Could you check a few things on this model? Use its own coordinates, in mm. A direction names the side the tool comes from. Give positions to 0.01 mm unless a question says otherwise; leave off trailing zeros. Write each loop counter-clockwise with the first axis right and the second up, starting at its lowest first coordinate (ties: lowest second). Pieces come first, ordered by that corner, then holes. Notation, with made-up numbers: M 19,87.5 L 67,87.5 A18 ccw 67,121.5 Z; hole C 13.25,79.25 d5. An arc over 180 degrees is marked long. Answer as CSV lines item,"result". Start each with the question number.
from build123d import *

# Parameters (mm, degrees)
F0_W      = 89.74328
F0_H      = 89.74328
F1_DEPTH  = 112.649
F3_DEPTH  = 8.382
F5_DEPTH  = 10.16
F7_DEPTH  = 10.16
F9_DEPTH  = 25.4
F10_R     = 25.4
F11_DEPTH = 12.7
F12_R     = 19.05
F13_DEPTH = 12.7
F14_R     = 12.7
F15_DEPTH = 42.97172


# Not quite as in the source:
# - a fillet or chamfer that OpenCascade refuses, or shapes differently, is made with other operations: its cross-section is extruded or revolved along the edge and cut away or added


with BuildPart() as f1:
    # F0 (on Right) → F1 (new body)
    with BuildSketch(Plane.YZ):
        with Locations((-0.1941993833, -7.4997466138)):
            Rectangle(F0_W, F0_H)
    extrude(amount=F1_DEPTH)

    # F2 (on face) → F3 (cut)
    with BuildSketch(Plane.XZ.offset(45.0658393833)):
        with BuildLine():
            ThreePointArc((103.9495, 19.7087333862), (103.0195640303, 21.9537974165), (100.7745, 22.8837333862))
            Line((100.7745, 22.8837333862), (11.8745, 22.8837333862))
            ThreePointArc((11.8745, 22.8837333862), (9.6294359697, 21.9537974165), (8.6995, 19.7087333862))
            Line((8.6995, 19.7087333862), (8.6995, 5.9419333862))
            ThreePointArc((8.6995, 5.9419333862), (9.6294359697, 3.6968693559), (11.8745, 2.7669333862))
            Line((11.8745, 2.7669333862), (100.7745, 2.7669333862))
            ThreePointArc((100.7745, 2.7669333862), (103.0195640303, 3.6968693559), (103.9495, 5.9419333862))
            Line((103.9495, 5.9419333862), (103.9495, 19.7087333862))
        make_face()
    extrude(amount=-F3_DEPTH, mode=Mode.SUBTRACT)

    # F4 (on face) → F5 (cut)
    with BuildSketch(Plane.XZ.offset(36.6838393833)):
        with BuildLine():
            ThreePointArc((8.6995, 8.0628333862), (9.6294359697, 5.8177693559), (11.8745, 4.8878333862))
            Line((11.8745, 4.8878333862), (100.7745, 4.8878333862))
            ThreePointArc((100.7745, 4.8878333862), (103.0195640303, 5.8177693559), (103.9495, 8.0628333862))
            Line((103.9495, 8.0628333862), (103.9495, 17.5878333862))
            ThreePointArc((103.9495, 17.5878333862), (103.0195640303, 19.8328974165), (100.7745, 20.7628333862))
            Line((100.7745, 20.7628333862), (11.8745, 20.7628333862))
            ThreePointArc((11.8745, 20.7628333862), (9.6294359697, 19.8328974165), (8.6995, 17.5878333862))
            Line((8.6995, 17.5878333862), (8.6995, 8.0628333862))
        make_face()
    extrude(amount=-F5_DEPTH, mode=Mode.SUBTRACT)

    # F6 (on face) → F7 (cut)
    with BuildSketch(Plane.XZ.offset(26.5238393833)):
        with BuildLine():
            ThreePointArc((16.637, 11.9363333862), (17.5669359697, 9.6912693559), (19.812, 8.7613333862))
            Line((19.812, 8.7613333862), (92.837, 8.7613333862))
            ThreePointArc((92.837, 8.7613333862), (95.0820640303, 9.6912693559), (96.012, 11.9363333862))
            Line((96.012, 11.9363333862), (96.012, 13.7143333862))
            ThreePointArc((96.012, 13.7143333862), (95.0820640303, 15.9593974165), (92.837, 16.8893333862))
            Line((92.837, 16.8893333862), (19.812, 16.8893333862))
            ThreePointArc((19.812, 16.8893333862), (17.5669359697, 15.9593974165), (16.637, 13.7143333862))
            Line((16.637, 13.7143333862), (16.637, 11.9363333862))
        make_face()
    extrude(amount=-F7_DEPTH, mode=Mode.SUBTRACT)

    # F8 (on face) → F9 (cut)
    with BuildSketch(Plane.XZ.offset(16.3638393833)):
        with BuildLine():
            ThreePointArc((88.9, 12.8253333862), (87.9700640303, 15.0703974165), (85.725, 16.0003333862))
            Line((85.725, 16.0003333862), (69.85, 16.0003333862))
            ThreePointArc((69.85, 16.0003333862), (67.6049359697, 15.0703974165), (66.675, 12.8253333862))
            ThreePointArc((66.675, 12.8253333862), (67.6049359697, 10.5802693559), (69.85, 9.6503333862))
            Line((69.85, 9.6503333862), (85.725, 9.6503333862))
            ThreePointArc((85.725, 9.6503333862), (87.9700640303, 10.5802693559), (88.9, 12.8253333862))
        make_face()
    extrude(amount=-F9_DEPTH, mode=Mode.SUBTRACT)

    # F10 (on face) → F11 (cut)
    with BuildSketch(Plane(origin=(0, 0, -52.3713866138), x_dir=(1, 0, 0), z_dir=(0, 0, -1))):
        with Locations((77.7875, -6.5774406167)):
            Circle(F10_R)
    extrude(amount=-F11_DEPTH, mode=Mode.SUBTRACT)

    # F12 (on face) → F13 (cut)
    with BuildSketch(Plane(origin=(0, 0, -39.6713866138), x_dir=(1, 0, 0), z_dir=(0, 0, -1))):
        with Locations((77.7875, -6.5774406167)):
            Circle(F12_R)
    extrude(amount=-F13_DEPTH, mode=Mode.SUBTRACT)

    # F14 (on face) → F15 (cut)
    with BuildSketch(Plane(origin=(0, 0, -26.9713866138), x_dir=(1, 0, 0), z_dir=(0, 0, -1))):
        with Locations((77.7875, -6.5774406167)):
            Circle(F14_R)
    extrude(amount=-F15_DEPTH, mode=Mode.SUBTRACT)

    # F16: fillet of radius 12.90574 on 2 edges, made by hand

    # F16_s1 → F16_t2 (revolve)
    with BuildSketch(Plane.XZ.offset(-6.5774406167)):
        with BuildLine():
            ThreePointArc((103.1875, -50.7880586878), (101.4881153597, -44.3868303291), (96.8375, -39.6713866138))
            Line((96.8375, -39.6713866138), (96.9686148, -39.4490531723))
            ThreePointArc((96.9686148, -39.4490531723), (100.0125, -39.4132718138), (103.1875, -39.4132718138))
            Line((103.1875, -39.4132718138), (103.4456148, -39.6713866138))
            Line((103.4456148, -39.6713866138), (103.4456148, -50.7880586878))
            Line((103.4456148, -50.7880586878), (103.1875, -50.7880586878))
        make_face()
    revolve(axis=Axis((77.7875, 6.5774406167, -39.6713866138), (0, 0, -1)))

    # F16_s3 → F16_t4 (revolve)
    with BuildSketch(Plane.XZ.offset(-6.5774406167)):
        with BuildLine():
            ThreePointArc((96.8375, -38.0880586878), (95.1381153597, -31.6868303291), (90.4875, -26.9713866138))
            Line((90.4875, -26.9713866138), (90.6186148, -26.7490531723))
            ThreePointArc((90.6186148, -26.7490531723), (93.6625, -26.7132718138), (96.8375, -26.7132718138))
            Line((96.8375, -26.7132718138), (97.0956148, -26.9713866138))
            Line((97.0956148, -26.9713866138), (97.0956148, -38.0880586878))
            Line((97.0956148, -38.0880586878), (96.8375, -38.0880586878))
        make_face()
    revolve(axis=Axis((77.7875, 6.5774406167, -26.9713866138), (0, 0, -1)))


solid = f1.part
1. On a 3-axis mill with a long thin cutter (end or side, diameter ignored), from which of +Z, -Z, +X, -X, +Y, -Y can I reach the whole of each face in a straight line? I mean faces 1 (the flat face through (56, 44.677, -8)), 2 (the cylindrical face through (9.7, -31.7, 19.9)). Say none if no direction works.
2. Thinking about a two-plate mould opening in Y: for faces 3 (the flat face through (56, -36.684, 4)), 4 (the cylindrical face through (17.54, -21.51, 9.72)), 5 (the flat face through (78, 1, 16)), 6 (the cylindrical face through (83.648, 17.845, -5.786)), which applies, pulls with the +Y half, pulls with the -Y half, needs draft (parallel to the pull), parting line crosses it, or undercut?
3. Please list where these lines run through material, in increasing order: line 1 (X direction, y = 16.5, z = -15); line 2 (Y direction, x = 21.5, z = 10.5); line 3 (X direction, y = -28, z = 16.5).
4. Will these pins go through, and if not, where does the flat tip stop? P1, Ø2.5, axis at x = 33, z = 20.5, coming from the -Y side; P2, Ø6.5, axis at x = 38, z = 11.5, coming from the -Y side; P3, Ø20.5, axis at x = 83, y = 9.5, coming from the -Z side.
5. Imagine slicing it at B-B, the plane z = -17. Please give me the cut outline in (x, y), plus the area to 3 significant figures.
Solutions:
1,face 1,"+Z, -Z, +X, -X, +Y"
1,face 2,"-Y"
2,face 3,"pulls with the -Y half"
2,face 4,"needs draft"
2,face 5,"undercut"
2,face 6,"undercut"
3,line 1,"0 to 69.86, 85.71 to 112.65"
3,line 2,"-16.36 to 44.68"
3,line 3,"0 to 8.7, 103.95 to 112.65"
4,P1,"y = -36.68"
4,P2,"y = -26.52"
4,P3,"z = -30.03"
5,outline,"M 0,-45.07 L 112.65,-45.07 L 112.65,44.68 L 0,44.68 Z; hole C 77.79,6.58 d25.4"
5,area,"9,600 mm²"
